Autodesk Inventor part; units mm, degrees
ref_plane "YZ Plane" through (0, 0, 0) normal (1, 0, 0) x (0, 1, 0)
ref_plane "XZ Plane" through (0, 0, 0) normal (0, 1, 0) x (-1, 0, 0)
ref_plane "XY Plane" through (0, 0, 0) normal (0, 0, 1) x (1, 0, 0)
sketch "Sketch1" plane through (0, 0, 0) normal (1, 0, 0) x (0, 1, 0)
  circle A0 centre (0, 0) radius 50
  dimension "d0" = 100
extrude "Extrusion1" add sketch "Sketch1" along normal mid plane 50
fillet "Fillet1" radius 5 2 edges at (-25, -50, 0) (25, -50, 0)
sketch "Sketch3" plane through (-25, 0, 0) normal (-1, 0, 0) x (0, 0, 1)
  circle A0 centre (0, 0) radius 25
  dimension "d11" = 50
extrude "Extrusion2" add sketch "Sketch3" along normal blind 5
sketch "Sketch4" plane through (-30, 0, 0) normal (-1, 0, 0) x (0, 0, 1)
  circle A0 centre (0, 0) radius 10
  dimension "d14" = 20
extrude "Extrusion3" add sketch "Sketch4" along normal blind 21.4
sketch "Sketch5" plane through (-51.4, 0, 0) normal (-1, 0, 0) x (0, 0, 1)
  circle A0 centre (0, 0) radius 50
hole "Hole2" at (-51.4, 0, 0) direction (1, 0, 0) diameter 15 end through all
sketch "Sketch6" plane through (0, 0, 0) normal (0, 1, 0) x (-1, 0, 0)
  circle A0 centre (41.2, 0) radius 3
  line L0 (51.4, -10) -> (51.4, 10)
  line L1 (41.2, 0) -> (51.4, 0) construction
  point P0 (0, 0)
  dimension "d24" = 6
  dimension "d25" = 10.2
extrude "Extrusion4" cut sketch "Sketch6" along normal blind 21.4
thread "Thread1"
properties part number "100mm Mecanum StandIn" material "Rubber"
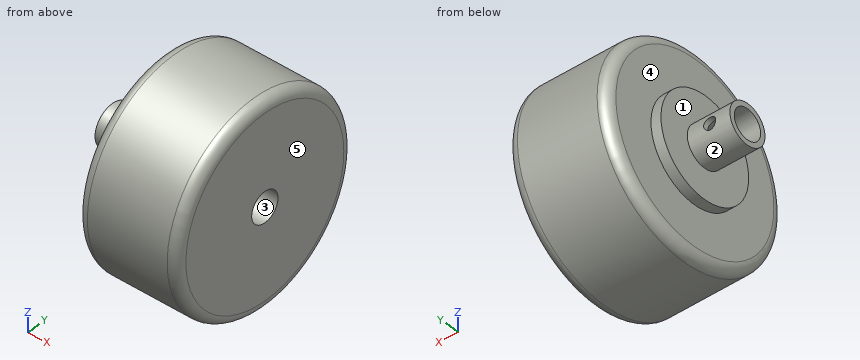
Can you work these out from the model? Positions are in its coordinate system, mm. Face numbers are marked on the shaded views. A direction names the side the tool comes from. Coordinates: 2 decimals unless noted, no trailing zeros. Loops run counter-clockwise (first coordinate to the right, second up) from the corner with the lowest first, then second, coordinate; pieces in that order, holes last.
Item 1: If we mould it in two halves opening along Y, with no side actions, what happens to the marked faces 1, 2 and 3? For each: released by +Y, released by -Y, zero draft, split by the parting line, or undercut.
Answers below:
face 1: zero draft
face 2: split by the parting line
face 3: undercut
Item 2: Please list where these lines run through material, in increasing order: L1, parallel to Z at x = -13.5, y = 0; L2, parallel to X at y = 9, z = 30.5; L3, parallel to X at y = 7.65, z = 0.
Answers below:
L1: z = -50 to -7.5, 7.5 to 50
L2: x = -25 to 25
L3: x = -51.4 to -44.2, -38.2 to 25
Item 3: Suppose I cut it at A-A (z = 0). Please give me the cut outline in (x, y).
Answers below:
outline: (-51.4, -10) - (-30, -10) - (-30, -25) - (-25, -25) - (-25, -45) arc R5 ccw to (-20, -50) - (20, -50) arc R5 ccw to (25, -45) - (25, -7.5) - (-51.4, -7.5) - close; (-51.4, 7.5) - (-44.2, 7.5) - (-44.2, 10) - (-51.4, 10) - close; (-38.2, 7.5) - (25, 7.5) - (25, 45) arc R5 ccw to (20, 50) - (-20, 50) arc R5 ccw to (-25, 45) - (-25, 25) - (-30, 25) - (-30, 10) - (-38.2, 10) - close
Item 4: I'm going to push flat-ended pins straight in: pin 1 (5 mm diameter, centred on x = -14.5, y = -29, fed in from -Z); pin 2 (8 mm diameter, centred on x = -41.2, z = 0, fed in from -Y); pin 3 (3 mm diameter, centred on x = 4.5, z = -13, fed in from -Y). Where does each tip first touch, or does it pass through?
Answers below:
pin 1: stops at z = -42.4
pin 2: stops at y = -10
pin 3: stops at y = -48.66
Item 5: Suppose I cut it at B-B (y = 0). Please give me the cut outline in (x, z).
Answers below:
outline: (-51.4, -10) - (-30, -10) - (-30, -25) - (-25, -25) - (-25, -45) arc R5 ccw to (-20, -50) - (20, -50) arc R5 ccw to (25, -45) - (25, -7.5) - (-51.4, -7.5) - close; (-51.4, 7.5) - (25, 7.5) - (25, 45) arc R5 ccw to (20, 50) - (-20, 50) arc R5 ccw to (-25, 45) - (-25, 25) - (-30, 25) - (-30, 10) - (-51.4, 10) - close
Item 6: Suppose I cut it at C-C (x = 7). Please give me the cut outline in (y, z).
Answers below:
outline: circle Ø100 at (0, 0); hole circle Ø15 at (0, 0)
Item 7: Suppose I cut it at D-D (x = -47). Please give me the cut outline in (y, z).
Answers below:
outline: circle Ø20 at (0, 0); hole circle Ø15 at (0, 0)
Item 8: Which directions (+Z, -Z, +X, -X, +Y, -Y) give clear straight access to the entire face, cutting with the end or side of a thin tool? Please do the marked faces 4 and 5.
Answers below:
face 4: -X
face 5: +Z, -Z, +X, +Y, -Y
